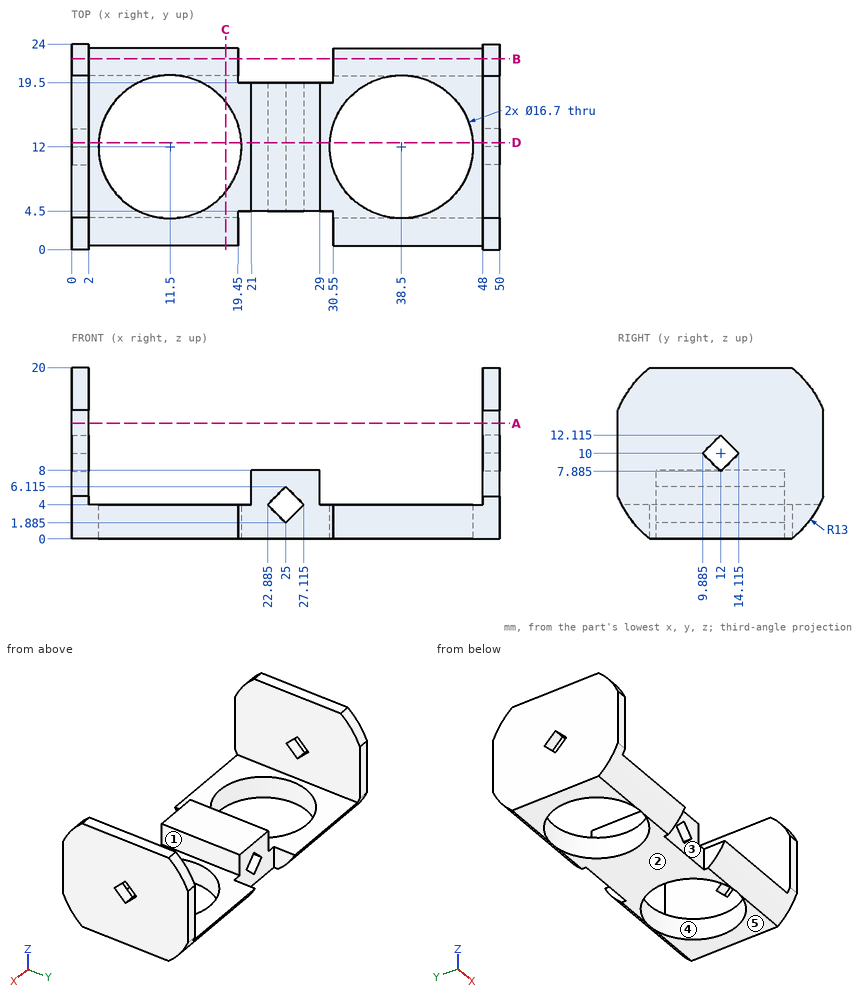
Check sheet for the drawn part. Datum: minimum x, y, z corner. Units: mm. A direction names the side the tool comes from. Round coordinates to 2 decimals unless told otherwise and drop trailing zeros. Order: outer loops, then holes, each group sorted by start corner. A loop starts at its lowest first (then second) coordinate and runs counter-clockwise, first axis right, second up.
1) Section check B-B (y = 22.25). Record the boundary of the cut face in (x, z).
2) Tool access check on the marked faces 1 and 2. Record the directions out of +Z, -Z, +X, -X, +Y, -Y that give a thin tool (end or side, any length) a straight path to the whole face; none if there is none.
3) Section check D-D (y = 12.5). Give the number of separate pieces and of enclosed holes in the cut face, and give its area (3 significant figures).
4) Mould release check, pull along Y, two halves, no side actions. Record for the marked faces 3, 4 and 5: +Y half, -Y half, draft (parallel to the pull), parting line (faces both ways), or undercut.
5) Section check A-A (z = 13.5). Record the boundary of the cut face in (x, y), and give its area (3 significant figures).
6) Scan lines: line 1 (X direction, y = 11.75, z = 7.5); line 2 (X direction, y = 16.75, z = 16.5); line 3 (Y direction, x = 28, z = 3.25). Record each from-to range of solid material in increasing order.
7) Go/stop test with flat-tipped pins: pin 1 Ø2.5 at (x, z) = (23, 2.5) entering from +Y; pin 2 Ø13.5 at (x, y) = (38.5, 12) entering from -Z; pin 3 Ø2.5 at (x, y) = (26.5, 15.5) entering from +Z. Record where each tip stops, or that it passes through.
8) Section check C-C (x = 18). Record the boundary of the cut face in (y, z).
Result:
1. outline: (0, 2) - (19.45, 2) - (19.45, 4) - (2, 4) - (2, 18) - (0, 18) - close; (30.55, 2) - (50, 2) - (50, 18) - (48, 18) - (48, 4) - (30.55, 4) - close
2. face 1: +Z, +Y, -Y
2. face 2: -Z, +X, -X, +Y, -Y
3. separate pieces: 5
3. enclosed holes: 1
3. area: 141 mm2
4. face 3: -Y half
4. face 4: undercut
4. face 5: draft
5. outline: (0, 0) - (2, 0) - (2, 24) - (0, 24) - close; (48, 0) - (50, 0) - (50, 24) - (48, 24) - close
5. area: 96.0 mm2
6. line 1: x = 0 to 2, 21 to 29, 48 to 50
6. line 2: x = 0 to 2, 48 to 50
6. line 3: y = 4.5 to 19.5
7. pin 1: stops at y = 19.5
7. pin 2: passes through
7. pin 3: stops at z = 8
8. outline: (0.47, 4) arc R13 ccw to (3.69, 0) - (6.76, 0) - (6.76, 4) - close; (17.24, 0) - (20.31, 0) arc R13 ccw to (23.53, 4) - (17.24, 4) - close
